Verification items for this drawing (mm, ordinates from the low corner). A direction names the side the tool comes from. Coordinates: 2 decimals unless noted, no trailing zeros. Write each loop counter-clockwise with the first axis right and the second up, starting at its lowest first coordinate (ties: lowest second). Pieces come first, ordered by that corner, then holes. Notation, with made-up numbers: M 72.5,-1 L 119.5,-1 A23 cw 119.5,7 Z; hole C -9.5,70 d6. An arc over 180 degrees is marked long. Write each question's results on one line, items separated by ' | '.
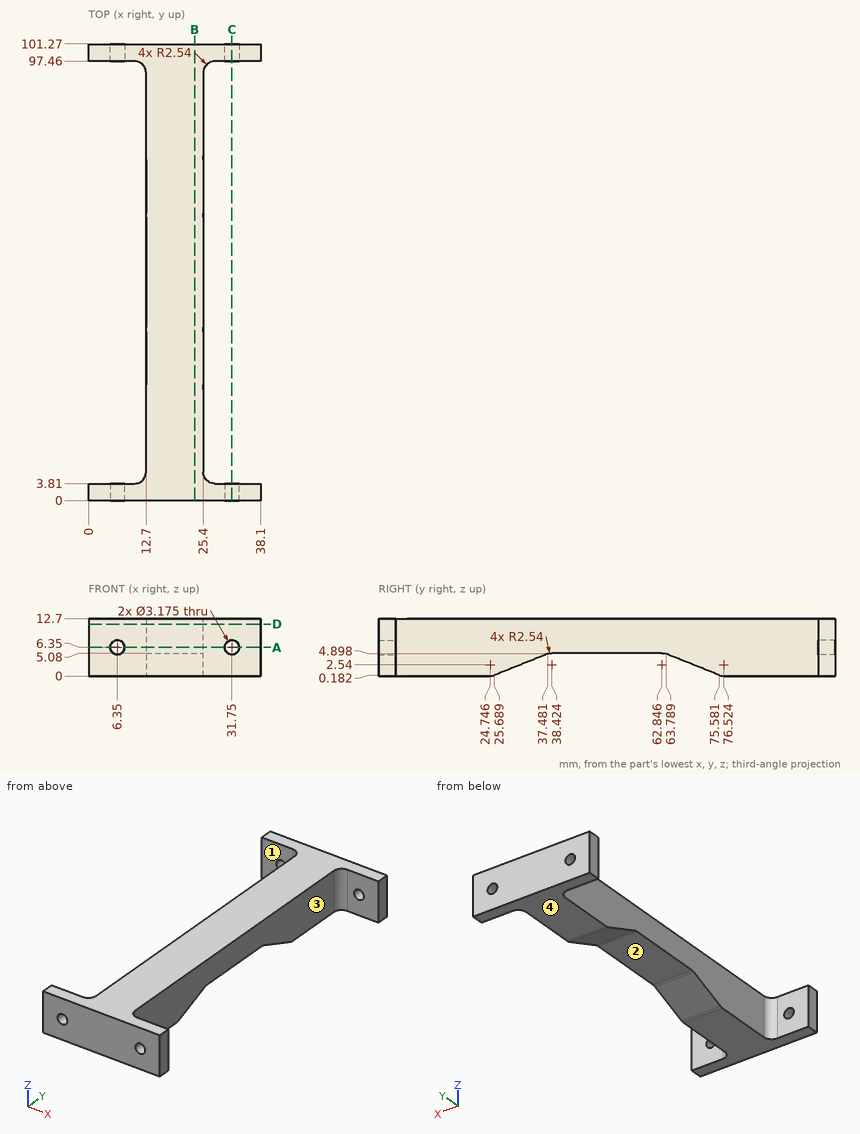
Q1. Scan lines: probe 1 along X at (y, z) = (99.25, 6.35); probe 2 along Y at (x, z) = (29.5, 11.25); probe 3 along Z at (x, y) = (31.75, 1.35). Record each from-to range of solid material in increasing order.
Geometry check:
probe 1: x = 0 to 4.76, 7.94 to 30.16, 33.34 to 38.1 | probe 2: y = 0 to 3.81, 97.46 to 101.27 | probe 3: z = 0 to 4.76, 7.94 to 12.7
Q2. Access from +Z, -Z, +X, -X, +Y, -Y to the whole of each face (thin tool, end or side, straight path). Record for the marked faces 1, 2, 3 and 4.
Geometry check:
face 1: +Z, -Z, -X | face 2: -Z, +X, -X | face 3: +Z, -Z, +X | face 4: -Z, +X, -X, +Y, -Y
Q3. Sectioned sample at B-B on x = 23.5. Record the cut outline in (y, z).
Geometry check:
outline: M 0,0 L 24.75,0 A2.54 ccw 25.69,0.18 L 37.48,4.9 A2.54 cw 38.42,5.08 L 62.85,5.08 A2.54 cw 63.79,4.9 L 75.58,0.18 A2.54 ccw 76.52,0 L 101.27,0 L 101.27,12.7 L 0,12.7 Z
Q4. Sectioned sample at D-D on z = 11.5. Record the cut outline in (x, y), and give its area (4 significant figures).
Geometry check:
outline: M 0,0 L 38.1,0 L 38.1,3.81 L 27.94,3.81 A2.54 cw 25.4,6.35 L 25.4,94.92 A2.54 cw 27.94,97.46 L 38.1,97.46 L 38.1,101.27 L 0,101.27 L 0,97.46 L 10.16,97.46 A2.54 cw 12.7,94.92 L 12.7,6.35 A2.54 cw 10.16,3.81 L 0,3.81 Z | area: 1,485 mm2
Q5. Depth check by flat-ended pin: P1, Ø1.9, axis at x = 31.75, z = 6.35, coming from the +Y side; P2, Ø6.5, axis at y = 43.5, z = 3.5, coming from the -X side; P3, Ø6.5, axis at x = 16, y = 55, coming from the -Z side; P4, Ø1.5, axis at y = 64, z = 6.5, coming from the +X side. Enter the tip coordinate at first touch or a pass-through.
Geometry check:
P1: passes through | P2: stops at x = 12.7 | P3: stops at z = 5.08 | P4: stops at x = 25.4
Q6. Sectioned sample at C-C on x = 31.75. Record the cut outline in (y, z).
Geometry check:
outline: M 0,0 L 3.81,0 L 3.81,4.76 L 0,4.76 Z; M 0,7.94 L 3.81,7.94 L 3.81,12.7 L 0,12.7 Z; M 97.46,0 L 101.27,0 L 101.27,4.76 L 97.46,4.76 Z; M 97.46,7.94 L 101.27,7.94 L 101.27,12.7 L 97.46,12.7 Z
Q7. Sectioned sample at A-A on z = 6.35. Give the number of separate pieces and of enclosed holes in the cut face, and give its area (3 significant figures).
Geometry check:
separate pieces: 5 | enclosed holes: 0 | area: 1,440 mm2
